Read the model definition and answer for the solid it produces. Units are mm, in the model's axes. A direction names the side the tool comes from. Round coordinates to 2 decimals unless told otherwise and drop trailing zeros. Order: outer loops, then holes, each group sorted by start corner. A loop starts at its lowest first (then second) coordinate and runs counter-clockwise, first axis right, second up.
from build123d import *

# Parameters (mm, degrees)
F1_DEPTH = 4
F2_R     = 2.05
F3_DEPTH = 34.001
F5_DEPTH = 1
F7_DEPTH = 1.5
F9_DEPTH = 1.501
F10_SIZE = 2
F11_R    = 3.99999


# Not quite as in the source:
# - a fillet or chamfer is up to 0.001 mm smaller than in the source, because OpenCascade refuses the exact size


with BuildPart() as f1:
    # F0 (on Front) → F1 (new body, symmetric)
    with BuildSketch(Plane.XZ):
        Polygon((15, 0), (0, 0), (-15, 0), (-15, 30), (-17, 30), (-17, -1.5), (0, -1.5), (17, -1.5), (17, 30), (15, 30), align=None)
    extrude(amount=F1_DEPTH, both=True)

    # F2 (on face) → F3 (cut, through all)
    with BuildSketch(Plane.YZ.offset(17)):
        with Locations((0, 25.95)):
            Circle(F2_R)
    extrude(amount=-F3_DEPTH, mode=Mode.SUBTRACT)

    # F4 (on Front) → F5 (join, symmetric)
    with BuildSketch(Plane.XZ):
        Polygon((-10, 0), (-15, 20), (-15, 0), align=None)
        Polygon((15, 20), (10, 0), (15, 0), align=None)
    extrude(amount=F5_DEPTH, both=True)

    # F6 (on face) → F7 (join, through all)
    with BuildSketch(Plane.XY):
        Polygon((15, -4), (-15, -4), (-17, -4), (-11.2264973081, -14), (0, -14), (11.2264973081, -14), (17, -4), align=None)
        Polygon((-11.2264973081, 14), (-17, 4), (-15, 4), (15, 4), (17, 4), (11.2264973081, 14), (0, 14), align=None)
    extrude(amount=-F7_DEPTH)

    # F8 (on face) → F9 (cut, through all)
    with BuildSketch(Plane.XY):
        Polygon((-7, -4), (-13.5358983849, -4), (-9.4944465005, -11), (9.4944465005, -11), (13.5358983849, -4), (7, -4), (7, 4), (13.5358983849, 4), (9.4944465005, 11), (-9.4944465005, 11), (-13.5358983849, 4), (-7, 4), align=None)
    extrude(amount=-F9_DEPTH, mode=Mode.SUBTRACT)

    # F10
    f10_edges = [f1.edges().sort_by_distance(p)[0] for p in [
        (-7, -4, -0.75),
        (-7, 4, -0.75),
        (7, -4, -0.75),
        (7, 4, -0.75),
    ]]
    chamfer(f10_edges, length=F10_SIZE)

    # F11 (radius 4 in the source; OpenCascade refuses exactly that, so slightly less here)
    f11_edges = [f1.edges().sort_by_distance(p)[0] for p in [
        (-16, -4, 30),
        (16, -4, 30),
        (16, 4, 30),
        (-16, 4, 30),
    ]]
    fillet(f11_edges, radius=F11_R)


solid = f1.part
Q1. A cutting plane is placed at B-B, the plane z = 12.5. Give the vertices of the cut face in (x, y) (3 decimals).
Outcome:
outline: (-17, -4) - (-15, -4) - (-15, -1) - (-13.125, -1) - (-13.125, 1) - (-15, 1) - (-15, 4) - (-17, 4) - close; (13.125, -1) - (15, -1) - (15, -4) - (17, -4) - (17, 4) - (15, 4) - (15, 1) - (13.125, 1) - close
Q2. A cutting plane is placed at D-D, the plane z = 25. Give the vertices of the cut face in (x, y), plus the area to 3 significant figures.
Outcome:
outline: (-17, -4) - (-15, -4) - (-15, -1.82) - (-17, -1.82) - close; (-17, 1.82) - (-15, 1.82) - (-15, 4) - (-17, 4) - close; (15, -4) - (17, -4) - (17, -1.82) - (15, -1.82) - close; (15, 1.82) - (17, 1.82) - (17, 4) - (15, 4) - close
area: 17.5 mm2
Q3. For a pull along Y with two mould halves and no side action, classify faces 1 (the face through (0, 14, -1)), 2 (the face through (8, 3, -1)), 3 (the face through (0, -14, -1)) as released by +Y, released by -Y, zero draft, split by the parting line, or undercut.
Outcome:
face 1: released by +Y
face 2: undercut
face 3: released by -Y
Q4. A cutting plane is placed at C-C, the plane y = -8. Give the vertices of the cut face in (x, z).
Outcome:
outline: (-14.69, -1.5) - (-11.23, -1.5) - (-11.23, 0) - (-14.69, 0) - close; (11.23, -1.5) - (14.69, -1.5) - (14.69, 0) - (11.23, 0) - close
Q5. A cutting plane is placed at A-A, the plane x = -8. Give the vertices of the cut face in (y, z).
Outcome:
outline: (-14, -1.5) - (-11, -1.5) - (-11, 0) - (-14, 0) - close; (-3, -1.5) - (3, -1.5) - (3, 0) - (-3, 0) - close; (11, -1.5) - (14, -1.5) - (14, 0) - (11, 0) - close
Q6. Straight lines are drawn through the part: probe 1 along X at (y, z) = (1.5, 24); probe 2 along Z at (x, y) = (-16.3, 0); probe 3 along Z at (x, y) = (4.5, -13). For each, find the intervals that lie inside material, in ascending order.
Outcome:
probe 1: x = -17 to -15, 15 to 17
probe 2: z = -1.5 to 23.9, 28 to 30
probe 3: z = -1.5 to 0
Q7. Flat-ended cylindrical pins translate along their axes: pin 1 (2 mm diameter, centred on x = 16, z = 15, fed in from +Y); pin 2 (5.5 mm diameter, centred on x = -12, z = 10.5, fed in from -Y); pin 3 (1.6 mm diameter, centred on x = 16.5, z = 10, fed in from -Y). Find the tip coordinate at first contact, or state that the pin passes through.
Outcome:
pin 1: stops at y = 4
pin 2: stops at y = -1
pin 3: stops at y = -4
Q8. For faces 4 (the face through (12.535, -0.014, 10.14)), 5 (the face through (0, -11, -1)), 6 (the face through (-14, 1, 6)), 7 (the face through (14, -1, 6)), 8 (the face through (15, -2, 15)), determine the directions among +Z, -Z, +X, -X, +Y, -Y from which every point of the face is accessible in a straight line to the end or side of a thin tool.
Outcome:
face 4: +Z, +Y, -Y
face 5: +Z, -Z
face 6: +Z, +Y
face 7: +Z, -Y
face 8: +Z
